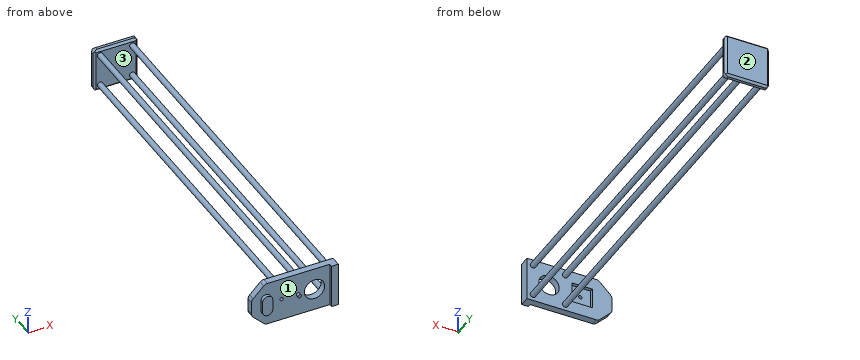
from build123d import *

# Parameters (mm, degrees)
SKETCH1_W            = 130
SKETCH1_H            = 130
BOSS_EXTRUDE2_DEPTH  = 20
SKETCH2_R            = 40
CUT_EXTRUDE1_DEPTH   = 95.074438611
SKETCH3_R            = 40
SKETCH3_R_2          = 30
BOSS_EXTRUDE3_DEPTH  = 20
SKETCH4_W            = 125.450553561
SKETCH4_H            = 31.465087356
CUT_EXTRUDE2_DEPTH   = 151.748134317
BOSS_EXTRUDE4_START  = -20
SKETCH5_R            = 40
SKETCH5_R_2          = 30
BOSS_EXTRUDE4_DEPTH  = 20
SKETCH6_R            = 8
BOSS_EXTRUDE5_DEPTH  = 1100
SKETCH7_W            = 130
SKETCH7_H            = 130
BOSS_EXTRUDE6_DEPTH  = 20
SKETCH8_W            = 20
SKETCH8_H            = 130
BOSS_EXTRUDE7_DEPTH  = 10
SKETCH9_W            = 130
SKETCH9_H            = 20
BOSS_EXTRUDE8_DEPTH  = 120
SKETCH10_R           = 5
BOSS_EXTRUDE9_DEPTH  = 10
SKETCH11_R           = 5
CUT_EXTRUDE3_DEPTH   = 1157.741111917
SKETCH12_W           = 60
SKETCH12_H           = 60
CUT_EXTRUDE4_DEPTH   = 10
CHAMFER1_SIZE        = 40
FILLET1_R            = 15
BOSS_EXTRUDE10_DEPTH = 10
CHAMFER2_SIZE        = 6
FILLET2_R            = 12


with BuildPart() as part:
    # Sketch1 → Boss-Extrude2 (new body)
    with BuildSketch(Plane(origin=(0, 0, 0), x_dir=(1, 0, 0), z_dir=(0, 1, 0))):
        Rectangle(SKETCH1_W, SKETCH1_H)
    extrude(amount=BOSS_EXTRUDE2_DEPTH)

    # Sketch2 → Cut-Extrude1 (cut, through all)
    with BuildSketch(Plane(origin=(0, 20, 0), x_dir=(1, 0, 0), z_dir=(0, 1, 0))):
        with Locations(Location((0, 0, 0), (0, 0, 270))):
            Circle(SKETCH2_R)
    extrude(amount=-CUT_EXTRUDE1_DEPTH, mode=Mode.SUBTRACT)

    # Sketch5 → Boss-Extrude4 (add)
    with BuildSketch(Plane.XZ.offset(BOSS_EXTRUDE4_START)):
        Circle(SKETCH5_R)
        with Locations(Location((0, 0, 0), (0, 0, 270))):
            Circle(SKETCH5_R_2, mode=Mode.SUBTRACT)
    extrude(amount=BOSS_EXTRUDE4_DEPTH)

    # Sketch6 → Boss-Extrude5 (add)
    with BuildSketch(Plane(origin=(0, 20, 0), x_dir=(1, 0, 0), z_dir=(0, 1, 0))):
        with Locations(Location((-47.32233047, 47.32233047, 0), (0, 0, 90))):
            Circle(SKETCH6_R)
        with Locations(Location((47.32233047, 47.32233047, 0), (0, 0, 90))):
            Circle(SKETCH6_R)
        with Locations(Location((47.32233047, -47.32233047, 0), (0, 0, 90))):
            Circle(SKETCH6_R)
        with Locations(Location((-47.32233047, -47.32233047, 0), (0, 0, 90))):
            Circle(SKETCH6_R)
    extrude(amount=BOSS_EXTRUDE5_DEPTH)

    # Sketch7 → Boss-Extrude6 (add)
    with BuildSketch(Plane(origin=(0, 1120, 0), x_dir=(1, 0, 0), z_dir=(0, 1, 0))):
        Rectangle(SKETCH7_W, SKETCH7_H)
    extrude(amount=BOSS_EXTRUDE6_DEPTH)

    # Sketch8 → Boss-Extrude7 (add)
    with BuildSketch(Plane.XZ):
        with Locations((55, 0)):
            Rectangle(SKETCH8_W, SKETCH8_H)
    extrude(amount=BOSS_EXTRUDE7_DEPTH)

    # Sketch9 → Boss-Extrude8 (add)
    with BuildSketch(Plane.ZY.offset(65)):
        with Locations((0, 10)):
            Rectangle(SKETCH9_W, SKETCH9_H)
    extrude(amount=BOSS_EXTRUDE8_DEPTH)

    # Sketch10 → Boss-Extrude9 (add)
    with BuildSketch(Plane.XZ):
        with Locations(Location((-48.62, 0, 0), (0, 0, 270))):
            Circle(SKETCH10_R)
    extrude(amount=BOSS_EXTRUDE9_DEPTH)

    # Sketch11 → Cut-Extrude3 (cut, through all)
    with BuildSketch(Plane.XZ):
        with Locations(Location((-97.24, 0, 0), (0, 0, 270))):
            Circle(SKETCH11_R)
    extrude(amount=-CUT_EXTRUDE3_DEPTH, mode=Mode.SUBTRACT)

    # Sketch12 → Cut-Extrude4 (cut)
    with BuildSketch(Plane(origin=(0, 20, 0), x_dir=(1, 0, 0), z_dir=(0, 1, 0))):
        with Locations((-97.24, 0)):
            Rectangle(SKETCH12_W, SKETCH12_H)
    extrude(amount=-CUT_EXTRUDE4_DEPTH, mode=Mode.SUBTRACT)

    # Chamfer1
    chamfer1_edges = [part.edges().sort_by_distance(p)[0] for p in [
        (-185, 10, -65),
        (-185, 10, 65),
    ]]
    chamfer(chamfer1_edges, length=CHAMFER1_SIZE)

    # Fillet1
    fillet1_edges = [part.edges().sort_by_distance(p)[0] for p in [
        (-185, 10, 25),
        (-185, 10, -25),
        (-145, 10, -65),
        (-145, 10, 65),
    ]]
    fillet(fillet1_edges, radius=FILLET1_R)

    # Sketch13 → Boss-Extrude10 (add)
    with BuildSketch(Plane.XZ):
        with BuildLine():
            Line((-157.902531243, -15.727314256), (-157.902531243, 15.727314256))
            ThreePointArc((-157.902531243, 15.727314256), (-142.902531243, 30.727314256), (-127.902531243, 15.727314256))
            Line((-127.902531243, 15.727314256), (-127.902531243, -15.727314256))
            ThreePointArc((-127.902531243, -15.727314256), (-142.902531243, -30.727314256), (-157.902531243, -15.727314256))
        make_face()
    extrude(amount=BOSS_EXTRUDE10_DEPTH)

    # Chamfer2
    chamfer2_edges = [part.edges().sort_by_distance(p)[0] for p in [
        (-65, 1120, 0),
        (0, 1120, 65),
        (65, 1120, 0),
        (0, 1120, -65),
        (-65, 1140, 0),
        (0, 1140, 65),
        (65, 1140, 0),
        (0, 1140, -65),
    ]]
    chamfer(chamfer2_edges, length=CHAMFER2_SIZE)

    # Fillet2
    fillet2_edges = [part.edges().sort_by_distance(p)[0] for p in [
        (-65, 1130, -65),
        (65, 1130, -65),
        (65, 1130, 65),
        (-65, 1130, 65),
    ]]
    fillet(fillet2_edges, radius=FILLET2_R)


with BuildPart() as body_2:
    # Sketch3 → Boss-Extrude3 (new body)
    with BuildSketch(Plane(origin=(0, 20, 0), x_dir=(1, 0, 0), z_dir=(0, 1, 0))):
        with Locations(Location((0, 0, 0), (0, 0, 270))):
            Circle(SKETCH3_R)
        with Locations(Location((0, 0, 0), (0, 0, 270))):
            Circle(SKETCH3_R_2, mode=Mode.SUBTRACT)
    extrude(amount=BOSS_EXTRUDE3_DEPTH)

    # Sketch4 → Cut-Extrude2 (cut, through all)
    with BuildSketch(Plane.XY.offset(65)):
        with Locations((-2.274723219, 35.732543678)):
            Rectangle(SKETCH4_W, SKETCH4_H)
    extrude(amount=-CUT_EXTRUDE2_DEPTH, mode=Mode.SUBTRACT)


solid = part.part
Design review of the part built by this model. Coordinates are the model's own, in mm. Face numbers are marked on the shaded views. Coordinates: 2 decimals unless noted, no trailing zeros. Order: outer loops, then holes, each group sorted by start corner. A loop starts at its lowest first (then second) coordinate and runs counter-clockwise, first axis right, second up.
Item 1: Take a section at A-A, the plane x = 0. Write out the cut boundary in (y, z).
Item 2: The part is to be moulded in two halves that separate along X. For the marked faces 1, 2 and 3, say which applies: pulls with the +X half, pulls with the -X half, needs draft (parallel to the pull), parting line crosses it, or undercut.
Item 3: Take a section at B-B, the plane y = 434.5. Write out the cut boundary in (x, z), then the cut area to 3 significant figures.
Item 4: For line 1 (X direction, y = 4.25, z = 0); line 2 (Z direction, x = 45.5, y = 405.5); line 3 (X direction, y = 297, z = -47), list the stretches that pass through material, from the lowest coordinate up.
Item 5: For pin 1 Ø4 at (y, z) = (1128.5, 22) entering from -X; pin 2 Ø5 at (y, z) = (-7, -2.5) entering from -X; pin 3 Ø4 at (x, z) = (-17, -48.5) entering from -Y, all flat-tipped, find the tip position at first contact; note any pin that passes through.
The answers:
1. outline: (0, -65) - (20, -65) - (20, -30) - (0, -30) - close; (0, 30) - (20, 30) - (20, 65) - (0, 65) - close; (1120, -59) - (1126, -65) - (1134, -65) - (1140, -59) - (1140, 59) - (1134, 65) - (1126, 65) - (1120, 59) - close
2. face 1: undercut
2. face 2: needs draft
2. face 3: undercut
3. outline: circle Ø16 at (-47.32, -47.32); circle Ø16 at (-47.32, 47.32); circle Ø16 at (47.32, -47.32); circle Ø16 at (47.32, 47.32)
3. area: 804 mm2
4. line 1: x = -185 to -102.24, -92.24 to -30, 30 to 65
4. line 2: z = -55.11 to -39.53, 39.53 to 55.11
4. line 3: x = -55.32 to -39.33, 39.33 to 55.32
5. pin 1: stops at x = -65
5. pin 2: stops at x = -157.9
5. pin 3: stops at y = 0
